```python
from build123d import *

# Parameters (mm, degrees)
F0_W     = 0.929184
F0_H     = 23.972953
F3_DEPTH = 1.016


with BuildPart() as f1:
    # F0 (on Top) → F1 (revolve)
    with BuildSketch(Plane.XY):
        with Locations((-62.214408, 0.097652)):
            Rectangle(F0_W, F0_H)
    revolve(axis=Axis((-61.749816, 0.848013, 0), (0, -1, 0)))

    # F2 (on face) → F3 (join)
    with BuildSketch(Plane(origin=(0, 12.084128, 0), x_dir=(-1, 0, 0), z_dir=(0, 1, 0))):
        with BuildLine():
            Line((68.013, 1.437184), (55.486632, 1.437184))
            ThreePointArc((55.486632, 1.437184), (54.768211, 1.139605), (54.470632, 0.421184))
            Line((54.470632, 0.421184), (54.470632, -0.421184))
            ThreePointArc((54.470632, -0.421184), (54.768211, -1.139605), (55.486632, -1.437184))
            Line((55.486632, -1.437184), (68.013, -1.437184))
            ThreePointArc((68.013, -1.437184), (68.731421, -1.139605), (69.029, -0.421184))
            Line((69.029, -0.421184), (69.029, 0.421184))
            ThreePointArc((69.029, 0.421184), (68.731421, 1.139605), (68.013, 1.437184))
        make_face()
    extrude(amount=-F3_DEPTH)


solid = f1.part
```
Model file for the job. Use its own axes, mm. A direction names the side the tool comes from. Round coordinates to 2 decimals unless told otherwise and drop trailing zeros. Order: outer loops, then holes, each group sorted by start corner. A loop starts at its lowest first (then second) coordinate and runs counter-clockwise, first axis right, second up. Notation, with made-up numbers: (37, 87.5) -> (60, 87.5) arc R19 ccw to (60, 92.5) -> close; hole circle Ø3 at (0, 41.5). An arc over 180 degrees is marked (long way). Use one line per item in the form item = value.
Item 1: Cut at A-A, the plane z = 0. Write the cut outline in (x, y).
Returned:
outline = (-69.03, 11.07) -> (-62.68, 11.07) -> (-62.68, -11.89) -> (-60.82, -11.89) -> (-60.82, 11.07) -> (-54.47, 11.07) -> (-54.47, 12.08) -> (-69.03, 12.08) -> close
Item 2: Drill centre lines: line 1 (Y direction, x = -63.5, z = 0.65); line 2 (X direction, y = -2, z = -0.05); line 3 (X direction, y = -10.25, z = 0.35). Where is each one in solid material? Low to high.
Returned:
line_1 = 11.07 to 12.08
line_2 = -62.68 to -60.82
line_3 = -62.61 to -60.89
Item 3: Flat gauge pins, fed straight in: pin 1 Ø1.5 at (x, z) = (-58, -1) entering from -Y; pin 2 Ø1 at (y, z) = (3, 0) entering from -X. Where does each tip first touch, or does it go through?
Returned:
pin_1 = 11.07
pin_2 = -62.68
Item 4: Cut at C-C, the plane y = -3. Write the cut outline in (x, z).
Returned:
outline = circle Ø1.86 at (-61.75, 0)
Item 5: Cut at D-D, the plane x = -59. Write the cut outline in (y, z), and give its area (3 significant figures).
Returned:
outline = (11.07, -1.44) -> (12.08, -1.44) -> (12.08, 1.44) -> (11.07, 1.44) -> close
area = 2.92 mm^2
Item 6: Tool access for faces 1 (the face through (-68.72, 11.58, -1.15)), 2 (the face through (-60.82, -0.25, -0.04)): list every direction of +Z, -Z, +X, -X, +Y, -Y with a clear straight run to the whole face (end or side of a thin tool).
Returned:
face_1 = -Z, -X, +Y, -Y
face_2 = -Y
Item 7: Cut at B-B, the plane x = -61.75. Write the cut outline in (y, z).
Returned:
outline = (-11.89, -0.93) -> (11.07, -0.93) -> (11.07, -1.44) -> (12.08, -1.44) -> (12.08, 1.44) -> (11.07, 1.44) -> (11.07, 0.93) -> (-11.89, 0.93) -> close
